Check sheet for the drawn part. Datum: minimum x, y, z corner. Units: mm. Round coordinates to 2 decimals unless told otherwise and drop trailing zeros. Order: outer loops, then holes, each group sorted by start corner. A loop starts at its lowest first (then second) coordinate and runs counter-clockwise, first axis right, second up. Notation, with made-up numbers: M 6.25,87 L 52.25,87 A28 ccw 52.25,118 Z; hole C 54,31.25 d3. An arc over 180 degrees is marked long. Use one line per item in the form item = value. Start each with the question number.
Item 1: Cross-section at C-C on y = 1.8. Enter the section's corners in (x, z).
Item 2: Cross-section at A-A on x = 8.25. Enter the section's corners in (y, z), then the cut area to 3 significant figures.
Item 3: Cross-section at D-D on z = 20. Enter the section's corners in (x, y).
Item 4: Thickness scan on probe 1 along Z at (x, y) = (4.5, 0.85); probe 2 along Z at (x, y) = (5.75, 1.6); probe 3 along X at (y, z) = (2.3, 20.5). Record the ranges inside material, lowest first. Write a range as [from, to].
Item 5: Go/stop test with flat-tipped pins: pin 1 Ø1 at (x, y) = (1.5, 1) entering from +Z; pin 2 Ø1.5 at (y, z) = (1.5, 7) entering from +X. Record where each tip stops, or that it passes through.
Item 6: Release check for a two-part mould opening along Z. For the marked faces 1, 2 and 3 record: +Z half, -Z half, draft (parallel to the pull), parting line (faces both ways), or undercut.
Item 7: Cross-section at B-B on x = 4. Enter the section's corners in (y, z), then the cut area to 3 significant figures.
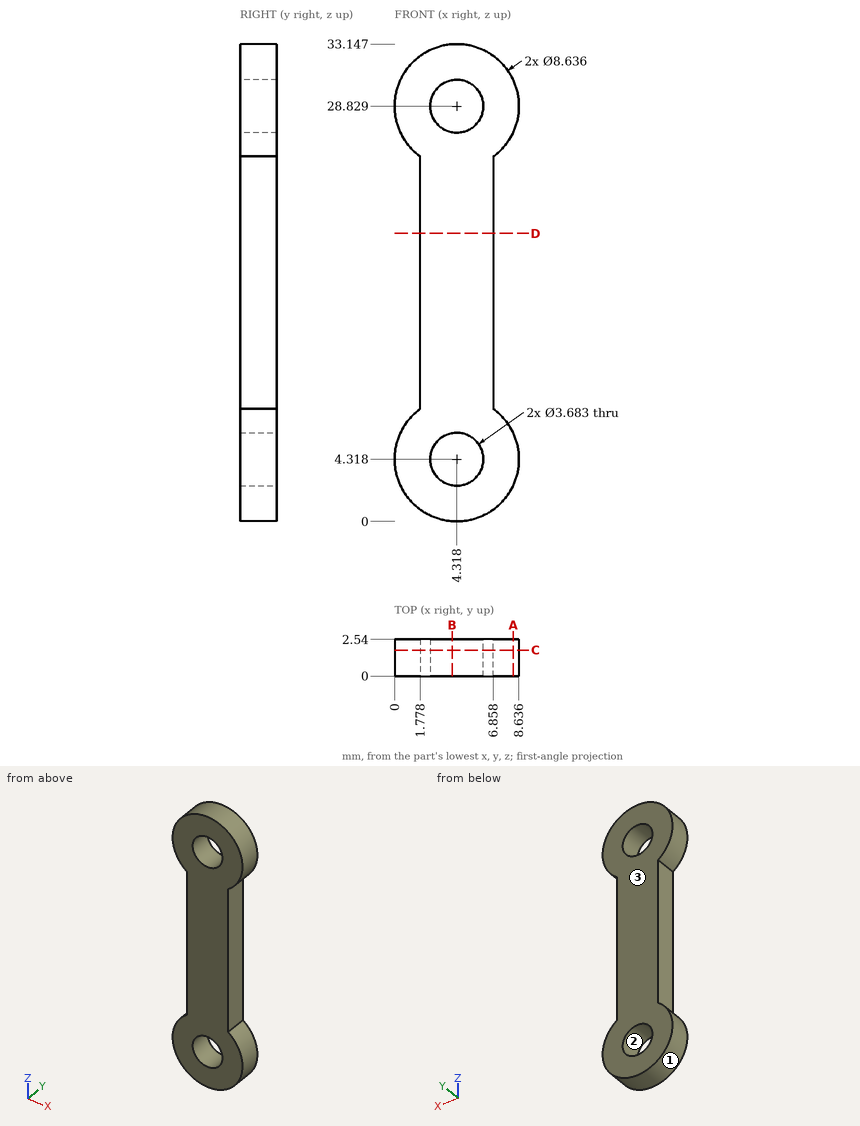
Output values:
q1.outline = M 1.78,7.81 A4.32 ccw long 6.86,7.81 L 6.86,25.34 A4.32 ccw long 1.78,25.34 Z; hole C 4.32,4.32 d3.68; hole C 4.32,28.83 d3.68
q2.outline = M 0,2.53 L 2.54,2.53 L 2.54,6.1 L 0,6.1 Z; M 0,27.04 L 2.54,27.04 L 2.54,30.61 L 0,30.61 Z
q2.area = 18.1 mm2
q3.outline = M 1.78,0 L 6.86,0 L 6.86,2.54 L 1.78,2.54 Z
q4.probe_1 = [0, 2.49], [6.15, 27], [30.66, 33.14]
q4.probe_2 = [0.24, 3.16], [5.48, 27.67], [29.99, 32.9]
q4.probe_3 = [1.78, 6.86]
q5.pin_1 = 32.47
q5.pin_2 = 8.18
q6.face_1 = undercut
q6.face_2 = undercut
q6.face_3 = draft
q7.outline = M 0,0.01 L 2.54,0.01 L 2.54,2.5 L 0,2.5 Z; M 0,6.13 L 2.54,6.13 L 2.54,27.02 L 0,27.02 Z; M 0,30.64 L 2.54,30.64 L 2.54,33.14 L 0,33.14 Z
q7.area = 65.7 mm2
